Autodesk Inventor part; units mm, degrees
ref_plane "YZ Plane" through (0, 0, 0) normal (1, 0, 0) x (0, 1, 0)
ref_plane "XZ Plane" through (0, 0, 0) normal (0, 1, 0) x (-1, 0, 0)
ref_plane "XY Plane" through (0, 0, 0) normal (0, 0, 1) x (1, 0, 0)
sketch "Sketch1" plane through (0, 0, 0) normal (0, 0, 1) x (1, 0, 0)
  line L0 (-750, 0) -> (750, 0) construction
  line L1 (750, 0) -> (750, -2700) construction
  line L2 (750, -2700) -> (-750, -2700) construction
  line L3 (-750, -2700) -> (-750, 0) construction
  line L4 (800, 50) -> (-800, 50) construction
  line L5 (-800, 50) -> (-800, -2750) construction
  line L6 (-800, -2750) -> (800, -2750) construction
  line L7 (800, -2750) -> (800, 50) construction
  line L8 (-850, 100) -> (850, 100) construction
  line L9 (850, 100) -> (850, -2800) construction
  line L10 (850, -2800) -> (-850, -2800) construction
  line L11 (-850, -2800) -> (-850, 100) construction
  arc A0 (750, 0) -> (745.2706, 0.6314) centre (0, -5600) ccw construction
  line L12 (-750, -2100) -> (750, -2100) construction
  line L13 (114.1118, -2698.3696) -> (750, -2100) construction
  arc A1 (750, -2100) -> (770.156, -238.4205) centre (-10250, -1050) ccw construction
  line L14 (750, 0) -> (749.6018, -2.9735) construction
  arc A2 (750, -3.0268) -> (0, 47) centre (-0.2, -5603) ccw construction
  line L15 (750, 0) -> (747.0136, -0.2851) construction
  arc A3 (767.1641, -238.6409) -> (747.4657, -5.0326) centre (-10252.9895, -1050.2527) ccw construction
  arc A4 (750.4522, -4.7486) -> (745.2706, 0.6314) centre (744.4791, -5.3162) ccw
  arc A5 (747.4657, -5.0326) -> (744.8748, -2.3426) centre (744.4792, -5.3164) ccw construction
  line L16 (750, -2100) -> (752.9864, -2100.2851) construction
  arc A6 (752.9864, -2100.2851) -> (771.2831, -213.263) centre (-10246.9891, -1050.0292) ccw construction
  line L17 (750, -2100) -> (752.0559, -2102.1848) construction
  line L18 (752.0559, -2102.1848) -> (752.0559, -2102.1848) construction
  arc A7 (749.1768, -2100.7746) -> (750.1074, -2098.8746) centre (747.1209, -2098.5898) ccw construction
  line L19 (0, -2697) -> (110, -2697) construction
  line L20 (112.0559, -2696.1848) -> (685.3133, -2156.7506) construction
  arc A8 (110, -2700) -> (114.1118, -2698.3696) centre (110, -2694) ccw construction
  arc A9 (110, -2697) -> (112.0559, -2696.1848) centre (110, -2694) ccw construction
  line L21 (685.3133, -2156.7506) -> (687.3692, -2158.9354) construction
  line L22 (752.0559, -2102.1848) -> (671.2185, -2178.2526) construction
  line L23 (671.2185, -2178.2526) -> (669.1626, -2176.0678) construction
  arc A10 (747.4657, -5.0326) -> (747.0136, -0.2851) centre (-10252.9895, -1050.2527) ccw construction
  arc A11 (745.2706, 0.6314) -> (0, 50) centre (0, -5600) ccw
  arc A12 (750.4522, -4.7486) -> (750, 0) centre (-10250, -1050) ccw construction
  line L24 (770.156, -238.4205) -> (767.1641, -238.6409) construction
  line L25 (768.2917, -213.4901) -> (771.2831, -213.263) construction
  arc A13 (770.156, -238.4205) -> (750.4522, -4.7486) centre (-10250, -1050) ccw
  line L26 (0, 100) -> (0, 50) construction
  line L27 (0, -2700) -> (0, -2697) construction
  line L28 (0, 47) -> (0, 0) construction
  line L29 (0, 50) -> (0, 47) construction
  arc A14 (752.0559, -2102.1848) -> (752.9864, -2100.2851) centre (749.9998, -2099.9999) ccw construction
  point P0 (0, -2750)
  dimension "d54" = 1500
  dimension "d55" = 2700
  dimension "d58" = 2100
  dimension "d68" = 6
  dimension "d70" = 3
  dimension "d75" = 3
  dimension "d83" = 6
  dimension "d86" = 3
  dimension "d112" = 239.271
  dimension "d113" = 50
  dimension "d114" = 50
  dimension "d115" = 3
  dimension "d117" = 110
  dimension "d118" = 25
  dimension "d119" = 111
  dimension "d120" = 25
contour flange "Contour Flange2" sketch "Sketch1" thickness 3 bend radius 3 width 910 along (0, 0, 1) mid plane no both sides no wall seen from (760.924, -121.5323, 0) lies toward (-0.9964637, -0.0840242, 0) curves A13 A4 A11
bend "Bend2"
corner "Corner2"
mirror "Mirror2" about plane through (0, 0, 0) normal (1, 0, 0)
equation "\"d36\" = Thickness"
equation "\"d37\" = BendReliefWidth"
equation "\"d38\" = BendReliefDepth"
equation "\"d39\" = MinimumRemnant"
equation "\"d40\" = TransitionRadius"
equation "\"d42\" = BendRadius"
equation "\"d44\" = CornerReliefSize"
equation "\"d45\" = GapSize"
equation "\"d46\" = JacobiRadiusSize"
equation "\"BendRadius\" = Thickness"
equation "\"BendReliefWidth\" = Thickness"
equation "\"BendReliefDepth\" = 0.5 * Thickness"
equation "\"CornerReliefSize\" = 4 * Thickness"
equation "\"MinimumRemnant\" = 2 * Thickness"
equation "\"TransitionRadius\" = BendRadius"
equation "\"JacobiRadiusSize\" = BendRadius"
equation "\"GapSize\" = Thickness"
properties part number "МОО 032 лист magic back-lowerback" material "Stainless Steel AISI 304"
The listing builds one solid part. Answer for the finished solid, in the listing's coordinates (mm). Coordinates: 2 decimals unless noted, no trailing zeros. Write each loop counter-clockwise with the first axis right and the second up, starting at its lowest first coordinate (ties: lowest second). Pieces come first, ordered by that corner, then holes. Notation, with made-up numbers: (74, -17.5) - (112, -17.5) arc R17 ccw to (112, 3.5) - close; hole circle Ø11 at (14.25, -20.75). An arc over 180 degrees is marked (long way). Return JSON: item names as keys, results as strings. Group by question number.
1. A cutting plane is placed at C-C, the plane y = -214. Determine the outline of the cut face in (x, z), plus the area to 3 significant figures.
2. A cutting plane is placed at B-B, the plane z = 473.5. Determine the outline of the cut face in (x, y), plus the area to 3 significant figures.
3. A cutting plane is placed at D-D, the plane x = 434.5. Determine the outline of the cut face in (y, z), plus the area to 3 significant figures.
4. Determine the mould class of faces 1 (the cylindrical face through (757.797, -120.149, 448.63)), 2 (the cylindrical face through (-761.06, -123.17, 448.63)), 3 (the cylindrical face through (760.786, -119.897, 448.63)) for opening direction X: released by +X, released by -X, zero draft, split by the parting line, or undercut.
5. Straight lines are drawn through the part: L1, parallel to X at y = -159, z = 491.5; L2, parallel to X at y = -8.5, z = 672.5; L3, parallel to Y at x = 191, z = 251. For each, find the intervals that lie inside material, in ascending order.
6. A cutting plane is placed at A-A, the plane y = -28.5. Determine the outline of the cut face in (x, z), plus the area to 3 significant figures.
Ans:
{
 "1": {"outline": "(-768.33, 0) - (-765.32, 0) - (-765.32, 910) - (-768.33, 910) - close; (765.32, 0) - (768.33, 0) - (768.33, 910) - (765.32, 910) - close", "area": "5,480 mm²"},
 "2": {"outline": "(-770.16, -238.42) - (-767.16, -238.64) arc R11046.82 cw to (-747.47, -5.03) arc R3 cw to (-744.87, -2.34) arc R5646.99 cw to (0, 47) arc R5646.99 cw to (744.87, -2.34) arc R3 cw to (747.47, -5.03) arc R11046.82 cw to (767.16, -238.64) - (770.16, -238.42) arc R11049.82 ccw to (750.45, -4.75) arc R6 ccw to (745.27, 0.63) arc R5649.99 ccw to (0, 50) arc R5649.99 ccw to (-745.27, 0.63) arc R6 ccw to (-750.45, -4.75) arc R11049.82 ccw to start", "area": "5,930 mm²"},
 "3": {"outline": "(30.26, 0) - (33.27, 0) - (33.27, 910) - (30.26, 910) - close", "area": "2,740 mm²"},
 "4": {"face 1": "undercut", "face 2": "released by -X", "face 3": "released by +X"},
 "5": {"L1": "-764.02 to -761.01, 761.01 to 764.02", "L2": "-750.81 to -747.79, 747.79 to 750.81", "L3": "43.77 to 46.77"},
 "6": {"outline": "(-752.68, 0) - (-749.67, 0) - (-749.67, 910) - (-752.68, 910) - close; (749.67, 0) - (752.68, 0) - (752.68, 910) - (749.67, 910) - close", "area": "5,480 mm²"}
}
